Build history of the part. All positions in model axes, mm. Face numbers are marked on the shaded views. A direction names the side the tool comes from. Round coordinates to 2 decimals unless told otherwise and drop trailing zeros. Order: outer loops, then holes, each group sorted by start corner. A loop starts at its lowest first (then second) coordinate and runs counter-clockwise, first axis right, second up. Notation, with made-up numbers: (75.25, 57.5) -> (110.25, 57.5) arc R26 cw to (110.25, 75.5) -> close; hole circle Ø4 at (1, 27.25). An arc over 180 degrees is marked (long way). Answer as a JSON object with one key per item and string values.
from build123d import *

# Parameters (mm, degrees)
AUFSATZ_LINEAR_AUSTRAGEN1_DEPTH      = 4.5
SCHNITT_LINEAR_AUSTRAGEN1_REACH      = 13.122
SCHNITT_LINEAR_AUSTRAGEN1_END_RADIUS = 3
SKIZZE3_R                            = 1.55
SCHNITT_LINEAR_AUSTRAGEN2_DEPTH      = 12.97914868
SCHNITT_LINEAR_AUSTRAGEN2_DEPTH_BACK = 12.97914868
SKIZZE4_W                            = 6
SKIZZE4_H                            = 5
FASE1_SIZE                           = 0.5


with BuildPart() as part:
    # Skizze1 → Aufsatz-Linear austragen1 (new, symmetric)
    with BuildSketch(Plane.XY):
        with BuildLine():
            Line((-4.5, 6.5), (4.5, 6.5))
            Line((4.5, 6.5), (4.5, 0))
            ThreePointArc((4.5, 0), (4.347413024, -1.161895004), (3.9, -2.244994432))
            ThreePointArc((3.9, -2.244994432), (2.875834261, -2.520828693), (2.6, -1.496662955))
            ThreePointArc((2.6, -1.496662955), (0, 3), (-2.6, -1.496662955))
            ThreePointArc((-2.6, -1.496662955), (-2.875834261, -2.520828693), (-3.9, -2.244994432))
            ThreePointArc((-3.9, -2.244994432), (-4.347413024, -1.161895004), (-4.5, 0))
            Line((-4.5, 0), (-4.5, 6.5))
        make_face()
    extrude(amount=AUFSATZ_LINEAR_AUSTRAGEN1_DEPTH, both=True)

    # Schnitt-Linear austragen1: up to this cylinder (the profile starts outside it)
    schnitt_linear_austragen1_end = Plane(origin=(0, 0, 0), z_dir=(0, 0, -1)) * Cylinder(SCHNITT_LINEAR_AUSTRAGEN1_END_RADIUS, 33.244, mode=Mode.PRIVATE)
    # Skizze3 → Schnitt-Linear austragen1 (cut, up to the surface)
    with BuildSketch(Plane(origin=(0, 6.5, 0), x_dir=(1, 0, 0), z_dir=(0, 1, 0)), mode=Mode.PRIVATE) as schnitt_linear_austragen1_sk1:
        with Locations(Location((0, 0, 0), (0, 0, 270))):
            Circle(SKIZZE3_R)
    schnitt_linear_austragen1_tool1 = extrude(schnitt_linear_austragen1_sk1.sketch, amount=-SCHNITT_LINEAR_AUSTRAGEN1_REACH, mode=Mode.PRIVATE) - schnitt_linear_austragen1_end
    add(schnitt_linear_austragen1_tool1.solids().sort_by_distance((0, 6.5, 0))[0], mode=Mode.SUBTRACT)

    # Skizze4 → Schnitt-Linear austragen2 (cut, two sides: drawn at the far end of the back side and taken through both)
    with BuildSketch(Plane.XY.offset(4.5).offset(-SCHNITT_LINEAR_AUSTRAGEN2_DEPTH_BACK)):
        with Locations((0, 2.5)):
            Rectangle(SKIZZE4_W, SKIZZE4_H)
    extrude(amount=SCHNITT_LINEAR_AUSTRAGEN2_DEPTH + SCHNITT_LINEAR_AUSTRAGEN2_DEPTH_BACK, mode=Mode.SUBTRACT)

    # Fase1
    fase1_edges = [part.edges().sort_by_distance(p)[0] for p in [
        (0, 5, -1.55),
    ]]
    chamfer(fase1_edges, length=FASE1_SIZE)


solid = part.part
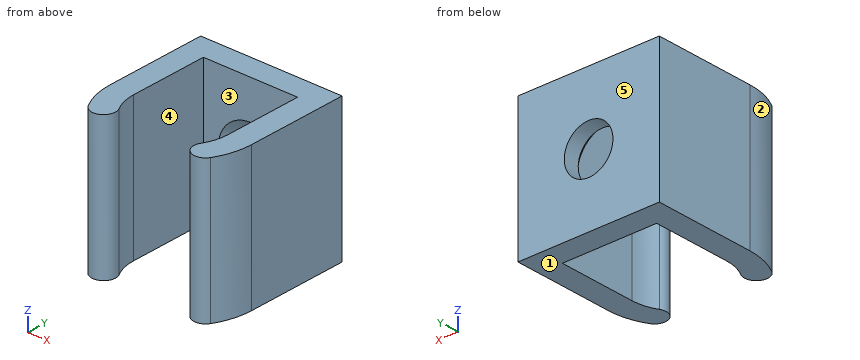
1) Flat gauge pin, fed straight in: pin 1 Ø3 at (x, z) = (0.5, 1) entering from -Y. Where does the tip first touch, or does it go through?
Checked values:
{"pin 1": "stops at y = 5"}
2) Pull direction X, two halves, no side cores. Call the marked faces 1, 2 and 3: pulls with the +X half, pulls with the -X half, needs draft (parallel to the pull), parting line crosses it, or undercut.
Checked values:
{"face 1": "needs draft", "face 2": "pulls with the -X half", "face 3": "undercut"}
3) Which spindle directions (+Z, -Z, +X, -X, +Y, -Y) get a long thin tool onto all of the face, cutting with end or side? Do the marked faces 4 and 5. Say none if no direction does.
Checked values:
{"face 4": "+Z, -Z", "face 5": "+Z, -Z, +X, -X, +Y"}
4) Probe L1, parallel to X at y = 5.8, z = 0; L2, parallel to X at y = 2.5, z = 1.75; L3, parallel to Y at x = -2, z = 1.5. List the from-to ranges inside material, lowest first. Write a range as from..to.
Checked values:
{"L1": "x = -4.5..-1.55, 1.55..4.5", "L2": "x = -4.5..-3, 3..4.5", "L3": "y = 5..6.5"}
5) Cut at D-D, the plane z = -2.5. Give the cut face in (x, y) (3 decimals), plus the area to 3 significant figures.
Checked values:
{"outline": "(-4.5, 0) arc R4.5 ccw to (-3.9, -2.245) arc R0.75 ccw to (-2.6, -1.497) arc R3 cw to (-3, 0) -> (-3, 5) -> (3, 5) -> (3, 0) arc R3 cw to (2.6, -1.497) arc R0.75 ccw to (3.9, -2.245) arc R4.5 ccw to (4.5, 0) -> (4.5, 6.5) -> (-4.5, 6.5) -> close", "area": "36.1 mm²"}
6) Cut at B-B, the plane x = 0. Give the cut face in (y, z), plus the area to 3 significant figures.
Checked values:
{"outline": "(5, -4.5) -> (6.5, -4.5) -> (6.5, -1.55) -> (5.5, -1.55) -> (5, -2.05) -> close; (5, 2.05) -> (5.5, 1.55) -> (6.5, 1.55) -> (6.5, 4.5) -> (5, 4.5) -> close", "area": "8.60 mm²"}
7) Cut at C-C, the plane y = 4.5. Give the cut face in (x, z), plus the area to 3 significant figures.
Checked values:
{"outline": "(-4.5, -4.5) -> (-3, -4.5) -> (-3, 4.5) -> (-4.5, 4.5) -> close; (3, -4.5) -> (4.5, -4.5) -> (4.5, 4.5) -> (3, 4.5) -> close", "area": "27.0 mm²"}
8) Cut at A-A, the plane z = 0. Give the cut face in (x, y) (3 decimals).
Checked values:
{"outline": "(-4.5, 0) arc R4.5 ccw to (-3.9, -2.245) arc R0.75 ccw to (-2.6, -1.497) arc R3 cw to (-3, 0) -> (-3, 5) -> (-2.05, 5) -> (-1.55, 5.5) -> (-1.55, 6.5) -> (-4.5, 6.5) -> close; (1.55, 5.5) -> (2.05, 5) -> (3, 5) -> (3, 0) arc R3 cw to (2.6, -1.497) arc R0.75 ccw to (3.9, -2.245) arc R4.5 ccw to (4.5, 0) -> (4.5, 6.5) -> (1.55, 6.5) -> close"}
